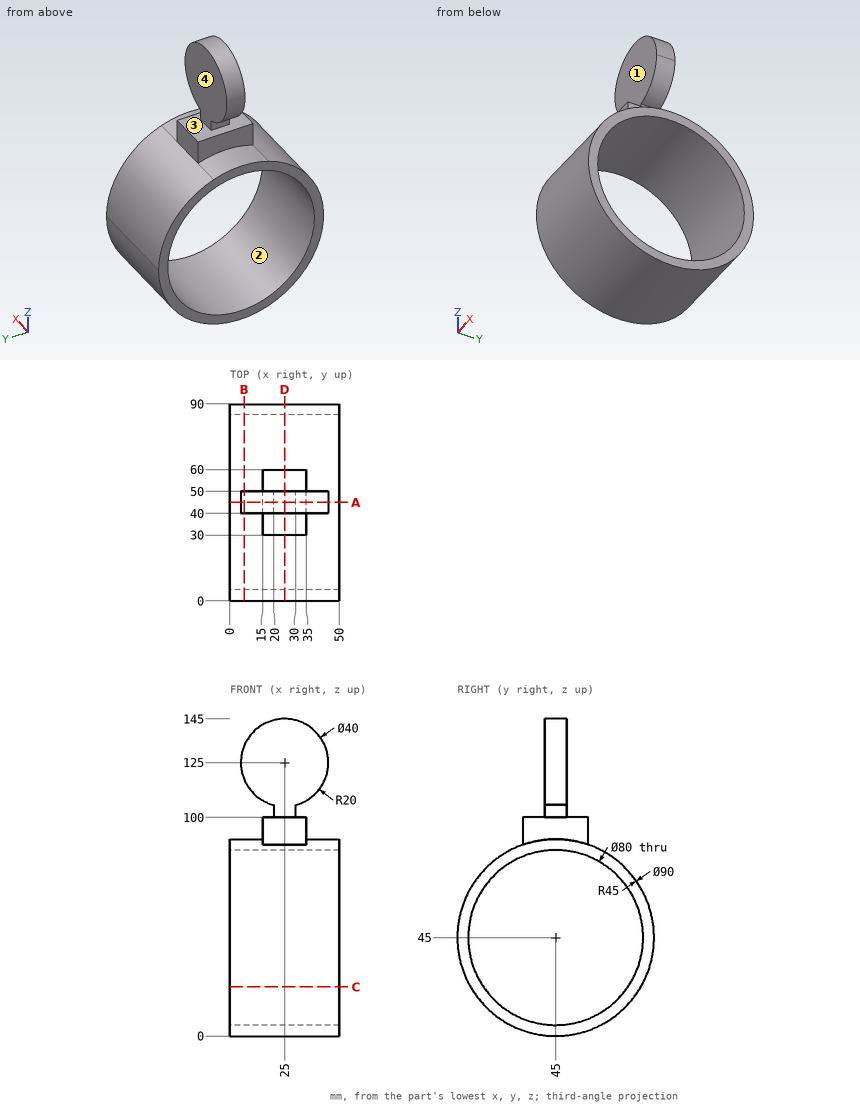
Drawing for the job (mm, zero at the part's lowest x, y, z). A direction names the side the tool comes from. Give positions to 0.01 mm unless a question says otherwise; leave off trailing zeros. Loops run counter-clockwise (first coordinate to the right, second up) from the corner with the lowest first, then second, coordinate; pieces in that order, holes last. Notation, with made-up numbers: (70, 31.5) - (92, 31.5) arc R20 cw to (92, 58.5) - close; hole circle Ø5 at (-27.5, -22). An arc over 180 degrees is marked (long way). Write item = value, one per line. Start each with the question number.
1) Band-saw the part on D-D on x = 25. Give the cut face in (y, z), plus the area to 3 significant figures.
2) Tool access for the marked faces 1 and 2: list every direction of +Z, -Z, +X, -X, +Y, -Y with a clear straight run to the whole face (end or side of a thin tool).
3) Drop flat-ended pins along their axis: pin 1 Ø4 at (x, y) = (27, 76) entering from +Z; pin 2 Ø16 at (x, y) = (26.5, 48.5) entering from +Z; pin 3 Ø6 at (y, z) = (45, 102) entering from +X; pin 4 Ø10 at (y, z) = (51.5, 90.5) entering from -X. Give the stop position or say it passes through.
4) Probe probe 1 along Y at (x, z) = (15.5, 45); probe 2 along Y at (x, z) = (25, 121.5); probe 3 along Z at (x, y) = (38, 45). List the from-to ranges inside material, lowest first. Write a range as from..to.
5) Band-saw the part on A-A on y = 45. Give the cut face in (x, z), plus the area to 3 significant figures.
6) Band-saw the part on C-C on z = 22.5. Give the cut face in (x, y).
7) Band-saw the part on B-B on x = 6.5. Give the cut face in (y, z).
8) Pull direction Z, two halves, no side cores. Call the marked faces 3 and 4: +Z half, -Z half, draft (parallel to the pull), parting line (faces both ways), or undercut.
Final values:
q1.outline = (30, 87.43) arc R45 ccw (long way) to (90, 45) arc R45 ccw to (60, 87.43) - (60, 100) - (50, 100) - (50, 145) - (40, 145) - (40, 100) - (30, 100) - close; hole circle Ø80 at (45, 45)
q1.area = 2,110 mm²
q2.face_1 = +Z, +X, -X, -Y
q2.face_2 = +X, -X
q3.pin_1 = 79.41
q3.pin_2 = 145
q3.pin_3 = 35
q3.pin_4 = 0
q4.probe_1 = 0..5, 85..90
q4.probe_2 = 40..50
q4.probe_3 = 0..5, 85..90, 109.8..140.2
q5.outline = (0, 0) - (50, 0) - (50, 5) - (0, 5) - close; (0, 85) - (50, 85) - (50, 90) - (35, 90) - (35, 100) - (30, 100) - (30, 105.64) arc R20 ccw (long way) to (20, 105.64) - (20, 100) - (15, 100) - (15, 90) - (0, 90) - close
q5.area = 2,010 mm²
q6.outline = (0, 6.03) - (50, 6.03) - (50, 11.93) - (0, 11.93) - close; (0, 78.07) - (50, 78.07) - (50, 83.97) - (0, 83.97) - close
q7.outline = (30, 87.43) arc R45 ccw (long way) to (90, 45) arc R45 ccw to (60, 87.43) arc R45 ccw to start; (40, 117.4) - (50, 117.4) - (50, 132.6) - (40, 132.6) - close; hole circle Ø80 at (45, 45)
q8.face_3 = undercut
q8.face_4 = draft
